from build123d import *

# Parameters (mm, degrees)
F0_R     = 9.525
F1_DEPTH = 7.9375
F2_SIZE2 = 2.54
F2_SIZE  = 2.54
F4_D     = 4.7625
F6_D     = 15.875
F6_DEPTH = 2.54
F6_TIP   = 4.7693311635


with BuildPart() as f1:
    # F0 (on Top) → F1 (new body)
    with BuildSketch(Plane.XY):
        Circle(F0_R)
    extrude(amount=F1_DEPTH)

    # F2
    f2_edges = [f1.edges().sort_by_distance(p)[0] for p in [
        (-9.525, 0, 7.9375),
    ]]
    chamfer(f2_edges, length=F2_SIZE, length2=F2_SIZE2)

    # F4 (through all)
    with Locations(Plane.XY.offset(7.9375)):
        with Locations((0, 0)):
            Hole(F4_D / 2)

    # F6
    with Locations(Plane(origin=(0, 0, 0), x_dir=(1, 0, 0), z_dir=(0, 0, -1))):
        with Locations((0, 0)):
            Hole(F6_D / 2, depth=F6_DEPTH)
            with Locations((0, 0, -(F6_DEPTH + F6_TIP / 2))):  # 118° drill point
                Cone(0, F6_D / 2, F6_TIP, mode=Mode.SUBTRACT)


solid = f1.part
Could you check a few things on this model? Use its own coordinates, in mm. Give positions to 0.01 mm unless a question says otherwise; leave off trailing zeros. Order: outer loops, then holes, each group sorted by start corner. A loop starts at its lowest first (then second) coordinate and runs counter-clockwise, first axis right, second up.
1. I need wall thicknesses on L1, parallel to Y at x = 0, z = 1.2 (1 decimal); L2, parallel to X at y = 5.25, z = 2.5; L3, parallel to Y at x = 2.25, z = 1.5. Which ranges of each line are inside material? Lowest first, please.
2. Will these pins go through, and if not, where does the flat tip stop? P1, Ø10, axis at x = -4, y = -4.5, coming from the -Z side; P2, Ø10, axis at x = 1.5, y = -0.5, coming from the -Z side (3 decimals); P3, Ø4, axis at y = 4.5, z = 1, coming from the -X side.
3. We'd pull the mould along X, two halves only. Please class faces 1 (the flat face through (3, 0, 7.938)), 2 (the cylindrical face through (1.72, 7.75, 1.29)), 3 (the cylindrical face through (-7.559, -5.796, 2.661)): pulls with the +X half, pulls with the -X half, needs draft (parallel to the pull), parting line crosses it, or undercut.
4. Suppose I cut it at B-B (z = 3.25). List the corners of the cut face in (x, y) for me (3 decimals).
5. Suppose I cut it at A-A (x = 0). List the corners of the cut face in (y, z) for me (1 decimal).
Solved:
1. L1: y = -9.5 to -7.9, 7.9 to 9.5
1. L2: x = -7.95 to -5.95, 5.95 to 7.95
1. L3: y = -9.26 to -7.61, 7.61 to 9.26
2. P1: stops at z = 0
2. P2: stops at z = 3.355
2. P3: stops at x = -9.19
3. face 1: needs draft
3. face 2: undercut
3. face 3: parting line crosses it
4. outline: circle Ø19.05 at (0, 0); hole circle Ø13.512 at (0, 0)
5. outline: (-9.5, 0) - (-7.9, 0) - (-7.9, 2.5) - (-2.4, 5.9) - (-2.4, 7.9) - (-7, 7.9) - (-9.5, 5.4) - close; (2.4, 5.9) - (7.9, 2.5) - (7.9, 0) - (9.5, 0) - (9.5, 5.4) - (7, 7.9) - (2.4, 7.9) - close
